Build history of the part. All positions in model axes, mm. A direction names the side the tool comes from. Round coordinates to 2 decimals unless told otherwise and drop trailing zeros. Loops run counter-clockwise (first coordinate to the right, second up) from the corner with the lowest first, then second, coordinate; pieces in that order, holes last. Notation, with made-up numbers: (15, 2.5) -> (28, 2.5) arc R12 cw to (28, 7.5) -> close; hole circle Ø9 at (-20.5, 32). An arc over 180 degrees is marked (long way). Put each result on its own line as item: value. Start each with the question number.
Item 1: Cut at B-B, the plane x = -160. List the corners of the cut face in (y, z), plus the area to 3 significant figures.
Item 2: Flat gauge pins, fed straight in: pin 1 Ø2 at (x, y) = (-53, 17.5) entering from +Z; pin 2 Ø21.5 at (x, y) = (-87.5, 16.5) entering from -Z; pin 3 Ø6 at (y, z) = (32, 13.5) entering from +X. Where does each tip first touch, or does it go through?
Item 3: Cut at A-A, the plane x = -12. List the corners of the cut face in (y, z).
Item 4: Drill centre lines: probe 1 along Z at (x, y) = (-25, 29); probe 2 along Z at (x, y) = (-148.5, 5.5); probe 3 along Y at (x, z) = (-160, -27). Where is each one in solid material? Low to high. Write a range as [from, to].
Item 5: Tool access for faces 1 (the flat face through (-14, 25, -35)), 2 (the cylindrical face through (-122.255, 24.65, -32.861)), 3 (the flat face through (-153, 25, 35)): list every direction of +Z, -Z, +X, -X, +Y, -Y with a clear straight run to the whole face (end or side of a thin tool).
Item 6: Cut at C-C, the plane y = 25. Count the separate pieces of the cut face and the enclosed holes in it, plus the area to 3 significant figures.
Item 7: Pull direction X, two halves, no side cores. Call faces 4 (the flat face through (-91, 25, -20)), 5 (the cylindrical face through (-180, 25, -30)), 6 (the flat face through (-25, 25, 45)): +X half, -X half, draft (parallel to the pull), parting line (faces both ways), or undercut.
Autodesk Inventor part; units mm, degrees
ref_plane "YZ Plane" through (0, 0, 0) normal (1, 0, 0) x (0, 1, 0)
ref_plane "XZ Plane" through (0, 0, 0) normal (0, 1, 0) x (-1, 0, 0)
ref_plane "XY Plane" through (0, 0, 0) normal (0, 0, 1) x (1, 0, 0)
sketch "Sketch1" plane through (0, 0, 0) normal (0, 1, 0) x (-1, 0, 0)
  line L0 (100, -45) -> (0, -45)
  line L1 (0, -45) -> (0, 0)
  line L2 (100, 45) -> (0, 45)
  line L3 (0, 45) -> (0, 0)
  line L4 (100, -45) -> (180, -45)
  line L5 (100, 45) -> (180, 45)
  line L6 (180, -45) -> (180, 45)
  dimension "d0" = 100
extrude "Extrusion1" add sketch "Sketch1" along normal blind 50
sketch "Sketch2" plane through (0, 50, 0) normal (0, 1, 0) x (1, 0, 0)
  line L0 (-180, -45) -> (0, -45)
  line L1 (-60, -45) -> (-60, 45)
  line L2 (0, 45) -> (-180, 45)
  line L3 (-120, 45) -> (-120, -45)
  line L4 (-60, 0) -> (-60, 20)
  line L5 (-60, 20) -> (-60, 0)
  line L6 (-60, 0) -> (-60, -20)
  line L7 (-60, -20) -> (-120, -20)
  line L8 (-60, 20) -> (-120, 20)
  line L9 (-180, -45) -> (0, -45)
  line L10 (0, 45) -> (-180, 45)
  line L11 (-180, 45) -> (-180, -45)
  line L12 (-180, -45) -> (-180, 45)
  line L13 (-180, -25) -> (-180, -15)
  line L14 (-180, 25) -> (-180, 15)
  line L15 (0, -45) -> (0, 45)
  line L16 (0, 45) -> (0, 35)
  line L17 (0, 35) -> (-60, 35)
  line L18 (0, -45) -> (0, -35)
  line L19 (0, -35) -> (-60, -35)
  line L20 (0, 0) -> (-20, 0)
  arc A0 (-0.6351, -35) -> (0, -34.641) centre (-20, 0) ccw
  arc A1 (0, 34.641) -> (-0.6351, 35) centre (-20, 0) ccw
  arc A2 (-39.3649, 35) -> (-39.3649, -35) centre (-20, 0) ccw
  line L21 (-120, 35) -> (-180, 35)
  line L22 (-120, -35) -> (-180, -35)
  line L23 (-180, 35) -> (-180, 25)
  line L24 (-180, 25) -> (-145, 25)
  line L25 (-180, -35) -> (-180, -25)
  line L26 (-180, -25) -> (-145, -25)
  arc A3 (-145, -25) -> (-145, 25) centre (-145, 0) ccw
  dimension "d5" = 60
  dimension "d13" = 20
  dimension "d14" = 20
  dimension "d18" = 10
  dimension "d19" = 10
  dimension "d25" = 10
  dimension "d26" = 10
  dimension "d27" = 20
  dimension "d28" = 10
  dimension "d29" = 10
extrude "Extrusion2" cut sketch "Sketch2" against normal blind 50 contours L11 L22 L3 L0 | L3 L7 L1 L0 | L11 L24 A3 L26 | A2 L17 A1 L15 A0 L19 | L3 L2 L1 L8 | L21 L11 L2 L3
fillet "Fillet1" radius 10 1 edges at (-39.3649, 25, 35)
fillet "Fillet2" radius 10 1 edges at (-39.3649, 25, -35)
fillet "Fillet3" radius 10 1 edges at (-60, 25, 45)
fillet "Fillet4" radius 10 3 edges at (-60, 25, 20) (-60, 25, -20) (-60, 25, -45)
fillet "Fillet5" radius 7.5 1 edges at (-120, 25, 35)
fillet "Fillet6" radius 7.5 3 edges at (-120, 25, 20) (-120, 25, -20) (-120, 25, -35)
sketch "Sketch3" plane through (-180, 0, -35) normal (0, 0, -1) x (-1, 0, 0)
  line L0 (0, 0) -> (0, 50)
  arc A0 (-8.775, 0) -> (-8.775, 50) centre (-40, 25) ccw
  line L1 (0, 50) -> (-52.5, 50)
  line L2 (0, 50) -> (-8.775, 50)
  line L3 (-8.775, 0) -> (0, 0)
  line L4 (0, 0) -> (0, 50)
  line L5 (-180, 0) -> (-180, 50)
  arc A1 (-171.225, 50) -> (-171.225, 0) centre (-140, 25) ccw
  line L6 (-130, 0) -> (-180, 0)
  line L7 (-180, 0) -> (-171.225, 0)
  line L8 (-171.225, 50) -> (-180, 50)
  line L9 (-180, 50) -> (-180, 0)
  point P0 (-180, 25)
  point P1 (-171.225, 0)
  point P2 (-8.775, 50)
  point P3 (0, 25)
extrude "Extrusion3" cut sketch "Sketch3" along normal mid plane 200
sketch "Sketch4" plane through (-50, 0, -45) normal (0, 0, -1) x (-1, 0, 0)
  arc A0 (-41.225, 50) -> (-41.225, 0) centre (-10, 25) ccw
  circle A1 centre (-30, 25) radius 2.5
  arc A2 (121.225, 0) -> (121.225, 50) centre (90, 25) ccw
  circle A3 centre (110, 25) radius 2.5
  point P0 (-50, 0)
  dimension "d44" = 5
  dimension "d46" = 5
extrude "Extrusion4" cut sketch "Sketch4" against normal blind 200
sketch "Sketch5" plane through (0, 0, 0) normal (0, -1, 0) x (1, 0, 0)
  point P0 (0, 0)
sketch "Sketch6" plane through (-127.5, 0, 35) normal (0, 0, 1) x (1, 0, 0)
  point P0 (127.5, 0)
properties part number "PartArm"
Reply:
1. outline: (0, -35) -> (22.5, -35) -> (22.5, -25) -> (0, -25) -> close; (0, 25) -> (22.5, 25) -> (22.5, 35) -> (0, 35) -> close; (27.5, -35) -> (50, -35) -> (50, -25) -> (27.5, -25) -> close; (27.5, 25) -> (50, 25) -> (50, 35) -> (27.5, 35) -> close
1. area: 900 mm^2
2. pin 1: stops at z = 44.8
2. pin 2: stops at z = -20
2. pin 3: stops at x = -56.44
3. outline: (0, -45) -> (50, -45) -> (50, -35) -> (0, -35) -> close; (0, 35) -> (50, 35) -> (50, 45) -> (0, 45) -> close
4. probe 1: z = [-45, -35], [35, 45]
4. probe 2: z = [-35, -25], [25, 35]
4. probe 3: y = [0, 22.5], [27.5, 50]
5. face 1: +Y, -Y
5. face 2: -Z, +Y, -Y
5. face 3: +Z, -X, +Y, -Y
6. separate pieces: 5
6. enclosed holes: 0
6. area: 5,290 mm^2
7. face 4: undercut
7. face 5: -X half
7. face 6: draft
